The model under review builds one solid part; all positions refer to its coordinate system, in mm. A direction names the side the tool comes from. Coordinates: 2 decimals unless noted, no trailing zeros. Loops run counter-clockwise (first coordinate to the right, second up) from the corner with the lowest first, then second, coordinate; pieces in that order, holes last. Notation, with made-up numbers: M 89.5,-18.75 L 98.5,-18.75 A20 ccw 98.5,19.25 Z; hole C -21,-30 d4. An arc over 180 degrees is marked long. Write item = value, one per line. Start each with the question number.
Q1. We need section B-B on x = 14. Give the boundary of the cut face in (y, z).
Q2. Wall thickness on probe 1 along X at (y, z) = (1.6, 161.5); probe 2 along X at (y, z) = (2.15, 94); probe 3 along X at (y, z) = (2.55, 109): over which ranges is each line inside the solid? List them lowest first.
Q3. For faces 1 (the face through (-97.659, 1.628, 4.365)), 2 (the face through (32.154, 1.628, -51.977)), list the 3-axis set-ups (+Z, -Z, +X, -X, +Y, -Y) from which the entire face can be reached by the end or side of a thin tool; tool diameter is ignored.
Q4. Mouldability with a two-part tool opening along X and no side actions: class faces 3 (the face through (-97.659, 1.628, -26.286)), 4 (the face through (32.154, 1.628, 125.823)) as released by +X, released by -X, zero draft, split by the parting line, or undercut.
Q5. We need section A-A on x = -2. Give the boundary of the cut face in (y, z), and give its area (3 significant figures).
Q6. We need section D-D on z = 0. Give the boundary of the cut face in (x, y).
Q7. We need section C-C on y = 0.95. Count the separate pieces of the cut face and the enclosed holes in it, and give its area (3 significant figures).
from build123d import *

# Parameters (mm, degrees)
SKETCH1_W           = 76.609890536
SKETCH1_H           = 190.5
SKETCH1_R           = 2.667
SKETCH1_R_2         = 3.436543353
BOSS_EXTRUDE1_DEPTH = 3.302


with BuildPart() as part:
    # Sketch1 → Boss-Extrude1 (new body)
    # profile 1 of 6: a face of its own
    with BuildSketch(Plane(origin=(0, 0, 0), x_dir=(1, 0, 0), z_dir=(0, 1, 0))):
        with Locations((-44.02898095, 106.210707771)):
            Rectangle(SKETCH1_W, SKETCH1_H)
    # profile 2 of 6: a face of its own
    with BuildSketch(Plane(origin=(0, 0, 0), x_dir=(1, 0, 0), z_dir=(0, 1, 0))):
        Polygon((-82.432035682, -192.239292229), (-5.724035682, -192.239292229), (-5.724035682, 10.960707771), (-82.333926218, 10.960707771), (-82.432035682, 10.862598307), align=None)
    # profile 3 of 6: a face of its own
    with BuildSketch(Plane(origin=(0, 0, 0), x_dir=(1, 0, 0), z_dir=(0, 1, 0))):
        Polygon((-113.420035682, -192.239292229), (-82.432035682, -192.239292229), (-82.432035682, 10.862598307), (-113.420035682, -20.125401693), align=None)
        with Locations(Location((-95.132035682, -185.889292229, 0), (0, 0, 90))):
            Circle(SKETCH1_R, mode=Mode.SUBTRACT)
        with Locations(Location((-95.132035682, -173.189292229, 0), (0, 0, 90))):
            Circle(SKETCH1_R, mode=Mode.SUBTRACT)
        with Locations(Location((-95.132035682, -160.489292229, 0), (0, 0, 90))):
            Circle(SKETCH1_R, mode=Mode.SUBTRACT)
        with Locations(Location((-95.132035682, -147.789292229, 0), (0, 0, 90))):
            Circle(SKETCH1_R, mode=Mode.SUBTRACT)
        with Locations(Location((-95.132035682, -135.089292229, 0), (0, 0, 90))):
            Circle(SKETCH1_R, mode=Mode.SUBTRACT)
        with Locations(Location((-95.132035682, -122.389292229, 0), (0, 0, 90))):
            Circle(SKETCH1_R, mode=Mode.SUBTRACT)
        with Locations(Location((-95.132035682, -109.689292229, 0), (0, 0, 90))):
            Circle(SKETCH1_R, mode=Mode.SUBTRACT)
        with Locations(Location((-95.132035682, -96.989292229, 0), (0, 0, 90))):
            Circle(SKETCH1_R, mode=Mode.SUBTRACT)
        with Locations(Location((-95.132035682, -84.289292229, 0), (0, 0, 90))):
            Circle(SKETCH1_R, mode=Mode.SUBTRACT)
        with Locations(Location((-95.132035682, -71.589292229, 0), (0, 0, 90))):
            Circle(SKETCH1_R, mode=Mode.SUBTRACT)
        with Locations(Location((-95.132035682, -58.889292229, 0), (0, 0, 90))):
            Circle(SKETCH1_R, mode=Mode.SUBTRACT)
        with Locations(Location((-95.132035682, -46.189292229, 0), (0, 0, 90))):
            Circle(SKETCH1_R, mode=Mode.SUBTRACT)
        with Locations(Location((-95.132035682, -33.489292229, 0), (0, 0, 90))):
            Circle(SKETCH1_R, mode=Mode.SUBTRACT)
        with Locations(Location((-95.132035682, -20.789292229, 0), (0, 0, 90))):
            Circle(SKETCH1_R, mode=Mode.SUBTRACT)
        with Locations(Location((-95.132035682, -8.089292229, 0), (0, 0, 90))):
            Circle(SKETCH1_R, mode=Mode.SUBTRACT)
    # profile 4 of 6: a face of its own
    with BuildSketch(Plane(origin=(0, 0, 0), x_dir=(1, 0, 0), z_dir=(0, 1, 0))):
        Polygon((44.242948133, -192.239292229), (44.242948133, -38.991111119), (-5.708870757, 10.960707771), (-5.724035682, 10.960707771), (-5.724035682, -192.239292229), align=None)
        with Locations(Location((6.904948133, -185.889292229, 0), (0, 0, 90))):
            Circle(SKETCH1_R_2, mode=Mode.SUBTRACT)
        with Locations(Location((6.904948133, -173.189292229, 0), (0, 0, 90))):
            Circle(SKETCH1_R_2, mode=Mode.SUBTRACT)
        with Locations(Location((6.904948133, -160.489292229, 0), (0, 0, 90))):
            Circle(SKETCH1_R_2, mode=Mode.SUBTRACT)
        with Locations(Location((6.904948133, -147.789292229, 0), (0, 0, 90))):
            Circle(SKETCH1_R_2, mode=Mode.SUBTRACT)
        with Locations(Location((32.304948133, -185.889292229, 0), (0, 0, 90))):
            Circle(SKETCH1_R_2, mode=Mode.SUBTRACT)
        with Locations(Location((32.304948133, -173.189292229, 0), (0, 0, 90))):
            Circle(SKETCH1_R_2, mode=Mode.SUBTRACT)
        with Locations(Location((32.304948133, -160.489292229, 0), (0, 0, 90))):
            Circle(SKETCH1_R_2, mode=Mode.SUBTRACT)
        with Locations(Location((32.304948133, -147.789292229, 0), (0, 0, 90))):
            Circle(SKETCH1_R_2, mode=Mode.SUBTRACT)
        with Locations(Location((6.904948133, -135.089292229, 0), (0, 0, 90))):
            Circle(SKETCH1_R_2, mode=Mode.SUBTRACT)
        with Locations(Location((6.904948133, -122.389292229, 0), (0, 0, 90))):
            Circle(SKETCH1_R_2, mode=Mode.SUBTRACT)
        with Locations(Location((6.904948133, -109.689292229, 0), (0, 0, 90))):
            Circle(SKETCH1_R_2, mode=Mode.SUBTRACT)
        with Locations(Location((6.904948133, -96.989292229, 0), (0, 0, 90))):
            Circle(SKETCH1_R_2, mode=Mode.SUBTRACT)
        with Locations(Location((32.304948133, -135.089292229, 0), (0, 0, 90))):
            Circle(SKETCH1_R_2, mode=Mode.SUBTRACT)
        with Locations(Location((32.304948133, -122.389292229, 0), (0, 0, 90))):
            Circle(SKETCH1_R_2, mode=Mode.SUBTRACT)
        with Locations(Location((32.304948133, -109.689292229, 0), (0, 0, 90))):
            Circle(SKETCH1_R_2, mode=Mode.SUBTRACT)
        with Locations(Location((32.304948133, -96.989292229, 0), (0, 0, 90))):
            Circle(SKETCH1_R_2, mode=Mode.SUBTRACT)
        with Locations(Location((6.904948133, -84.289292229, 0), (0, 0, 90))):
            Circle(SKETCH1_R_2, mode=Mode.SUBTRACT)
        with Locations(Location((6.904948133, -71.589292229, 0), (0, 0, 90))):
            Circle(SKETCH1_R_2, mode=Mode.SUBTRACT)
        with Locations(Location((6.904948133, -58.889292229, 0), (0, 0, 90))):
            Circle(SKETCH1_R_2, mode=Mode.SUBTRACT)
        with Locations(Location((6.904948133, -46.189292229, 0), (0, 0, 90))):
            Circle(SKETCH1_R_2, mode=Mode.SUBTRACT)
        with Locations(Location((32.304948133, -84.289292229, 0), (0, 0, 90))):
            Circle(SKETCH1_R_2, mode=Mode.SUBTRACT)
        with Locations(Location((32.304948133, -71.589292229, 0), (0, 0, 90))):
            Circle(SKETCH1_R_2, mode=Mode.SUBTRACT)
        with Locations(Location((32.304948133, -58.889292229, 0), (0, 0, 90))):
            Circle(SKETCH1_R_2, mode=Mode.SUBTRACT)
        with Locations(Location((32.304948133, -46.189292229, 0), (0, 0, 90))):
            Circle(SKETCH1_R_2, mode=Mode.SUBTRACT)
        with Locations(Location((6.904948133, -33.489292229, 0), (0, 0, 90))):
            Circle(SKETCH1_R_2, mode=Mode.SUBTRACT)
        with Locations(Location((6.904948133, -20.789292229, 0), (0, 0, 90))):
            Circle(SKETCH1_R_2, mode=Mode.SUBTRACT)
        with Locations(Location((6.904948133, -8.089292229, 0), (0, 0, 90))):
            Circle(SKETCH1_R_2, mode=Mode.SUBTRACT)
        with Locations(Location((32.304948133, -33.489292229, 0), (0, 0, 90))):
            Circle(SKETCH1_R_2, mode=Mode.SUBTRACT)
    # profile 5 of 6: a face of its own
    with BuildSketch(Plane(origin=(0, 0, 0), x_dir=(1, 0, 0), z_dir=(0, 1, 0))):
        Polygon((-5.724035682, 10.960707771), (-5.708870757, 10.960707771), (44.242948133, 60.912526661), (44.242948133, 201.460707771), (-5.724035682, 201.460707771), align=None)
        with Locations(Location((6.904948133, 30.010707771, 0), (0, 0, 90))):
            Circle(SKETCH1_R_2, mode=Mode.SUBTRACT)
        with Locations(Location((6.904948133, 42.710707771, 0), (0, 0, 90))):
            Circle(SKETCH1_R_2, mode=Mode.SUBTRACT)
        with Locations(Location((6.904948133, 55.410707771, 0), (0, 0, 90))):
            Circle(SKETCH1_R_2, mode=Mode.SUBTRACT)
        with Locations(Location((6.904948133, 68.110707771, 0), (0, 0, 90))):
            Circle(SKETCH1_R_2, mode=Mode.SUBTRACT)
        with Locations(Location((6.904948133, 80.810707771, 0), (0, 0, 90))):
            Circle(SKETCH1_R_2, mode=Mode.SUBTRACT)
        with Locations(Location((6.904948133, 93.510707771, 0), (0, 0, 90))):
            Circle(SKETCH1_R_2, mode=Mode.SUBTRACT)
        with Locations(Location((32.304948133, 55.410707771, 0), (0, 0, 90))):
            Circle(SKETCH1_R_2, mode=Mode.SUBTRACT)
        with Locations(Location((32.304948133, 68.110707771, 0), (0, 0, 90))):
            Circle(SKETCH1_R_2, mode=Mode.SUBTRACT)
        with Locations(Location((32.304948133, 80.810707771, 0), (0, 0, 90))):
            Circle(SKETCH1_R_2, mode=Mode.SUBTRACT)
        with Locations(Location((32.304948133, 93.510707771, 0), (0, 0, 90))):
            Circle(SKETCH1_R_2, mode=Mode.SUBTRACT)
        with Locations(Location((6.904948133, 106.210707771, 0), (0, 0, 90))):
            Circle(SKETCH1_R_2, mode=Mode.SUBTRACT)
        with Locations(Location((6.904948133, 118.910707771, 0), (0, 0, 90))):
            Circle(SKETCH1_R_2, mode=Mode.SUBTRACT)
        with Locations(Location((6.904948133, 131.610707771, 0), (0, 0, 90))):
            Circle(SKETCH1_R_2, mode=Mode.SUBTRACT)
        with Locations(Location((6.904948133, 144.310707771, 0), (0, 0, 90))):
            Circle(SKETCH1_R_2, mode=Mode.SUBTRACT)
        with Locations(Location((32.304948133, 106.210707771, 0), (0, 0, 90))):
            Circle(SKETCH1_R_2, mode=Mode.SUBTRACT)
        with Locations(Location((32.304948133, 118.910707771, 0), (0, 0, 90))):
            Circle(SKETCH1_R_2, mode=Mode.SUBTRACT)
        with Locations(Location((32.304948133, 131.610707771, 0), (0, 0, 90))):
            Circle(SKETCH1_R_2, mode=Mode.SUBTRACT)
        with Locations(Location((32.304948133, 144.310707771, 0), (0, 0, 90))):
            Circle(SKETCH1_R_2, mode=Mode.SUBTRACT)
        with Locations(Location((6.904948133, 157.010707771, 0), (0, 0, 90))):
            Circle(SKETCH1_R_2, mode=Mode.SUBTRACT)
        with Locations(Location((6.904948133, 169.710707771, 0), (0, 0, 90))):
            Circle(SKETCH1_R_2, mode=Mode.SUBTRACT)
        with Locations(Location((6.904948133, 182.410707771, 0), (0, 0, 90))):
            Circle(SKETCH1_R_2, mode=Mode.SUBTRACT)
        with Locations(Location((6.904948133, 195.110707771, 0), (0, 0, 90))):
            Circle(SKETCH1_R_2, mode=Mode.SUBTRACT)
        with Locations(Location((32.304948133, 157.010707771, 0), (0, 0, 90))):
            Circle(SKETCH1_R_2, mode=Mode.SUBTRACT)
        with Locations(Location((32.304948133, 169.710707771, 0), (0, 0, 90))):
            Circle(SKETCH1_R_2, mode=Mode.SUBTRACT)
        with Locations(Location((32.304948133, 182.410707771, 0), (0, 0, 90))):
            Circle(SKETCH1_R_2, mode=Mode.SUBTRACT)
        with Locations(Location((32.304948133, 195.110707771, 0), (0, 0, 90))):
            Circle(SKETCH1_R_2, mode=Mode.SUBTRACT)
    # profile 6 of 6: a face of its own
    with BuildSketch(Plane(origin=(0, 0, 0), x_dir=(1, 0, 0), z_dir=(0, 1, 0))):
        Polygon((-82.333926218, 10.960707771), (-113.420035682, 42.046817234), (-113.420035682, 201.460707771), (-82.333926218, 201.460707771), align=None)
        with Locations(Location((-95.132035682, 30.010707771, 0), (0, 0, 90))):
            Circle(SKETCH1_R, mode=Mode.SUBTRACT)
        with Locations(Location((-95.132035682, 42.710707771, 0), (0, 0, 90))):
            Circle(SKETCH1_R, mode=Mode.SUBTRACT)
        with Locations(Location((-95.132035682, 55.410707771, 0), (0, 0, 90))):
            Circle(SKETCH1_R, mode=Mode.SUBTRACT)
        with Locations(Location((-95.132035682, 68.110707771, 0), (0, 0, 90))):
            Circle(SKETCH1_R, mode=Mode.SUBTRACT)
        with Locations(Location((-95.132035682, 80.810707771, 0), (0, 0, 90))):
            Circle(SKETCH1_R, mode=Mode.SUBTRACT)
        with Locations(Location((-95.132035682, 93.510707771, 0), (0, 0, 90))):
            Circle(SKETCH1_R, mode=Mode.SUBTRACT)
        with Locations(Location((-95.132035682, 106.210707771, 0), (0, 0, 90))):
            Circle(SKETCH1_R, mode=Mode.SUBTRACT)
        with Locations(Location((-95.132035682, 118.910707771, 0), (0, 0, 90))):
            Circle(SKETCH1_R, mode=Mode.SUBTRACT)
        with Locations(Location((-95.132035682, 131.610707771, 0), (0, 0, 90))):
            Circle(SKETCH1_R, mode=Mode.SUBTRACT)
        with Locations(Location((-95.132035682, 144.310707771, 0), (0, 0, 90))):
            Circle(SKETCH1_R, mode=Mode.SUBTRACT)
        with Locations(Location((-95.132035682, 157.010707771, 0), (0, 0, 90))):
            Circle(SKETCH1_R, mode=Mode.SUBTRACT)
        with Locations(Location((-95.132035682, 169.710707771, 0), (0, 0, 90))):
            Circle(SKETCH1_R, mode=Mode.SUBTRACT)
        with Locations(Location((-95.132035682, 182.410707771, 0), (0, 0, 90))):
            Circle(SKETCH1_R, mode=Mode.SUBTRACT)
        with Locations(Location((-95.132035682, 195.110707771, 0), (0, 0, 90))):
            Circle(SKETCH1_R, mode=Mode.SUBTRACT)
    extrude(amount=BOSS_EXTRUDE1_DEPTH)


solid = part.part
Returned:
q1.outline = M 0,-201.46 L 3.3,-201.46 L 3.3,-30.67 L 0,-30.67 Z; M 0,8.75 L 3.3,8.75 L 3.3,192.24 L 0,192.24 Z
q2.probe_1 = -113.42 to -97.6, -92.66 to 3.62, 10.19 to 29.02, 35.59 to 44.24
q2.probe_2 = -113.42 to 5.21, 8.6 to 30.61, 34 to 44.24
q2.probe_3 = -113.42 to -97.71, -92.56 to 3.54, 10.27 to 28.94, 35.67 to 44.24
q3.face_1 = -X, +Y, -Y
q3.face_2 = +Y, -Y
q4.face_3 = released by -X
q4.face_4 = undercut
q5.outline = M 0,-201.46 L 3.3,-201.46 L 3.3,-14.67 L 0,-14.67 Z; M 0,-7.25 L 3.3,-7.25 L 3.3,192.24 L 0,192.24 Z
q5.area = 1,280 mm^2
q6.outline = M -93.29,0 L 5.25,0 L 5.25,3.3 L -93.29,3.3 Z
q7.separate_pieces = 1
q7.enclosed_holes = 83
q7.area = 56,000 mm^2
